from build123d import *

# Parameters (mm, degrees)
BOSS_EXTRUDE1_DEPTH = 127
SKETCH2_R           = 2.049999964
SKETCH2_W           = 19.05
SKETCH2_H           = 8.89
CUT_EXTRUDE1_DEPTH  = 25.48749992
FILLET1_R           = 12.7
BOSS_EXTRUDE2_REACH = 18.672
SKETCH4_W           = 1.891908828
SKETCH4_H           = 8.89


with BuildPart() as part:
    # Sketch1 → Boss-Extrude1 (new body)
    with BuildSketch(Plane(origin=(0, 0, 0), x_dir=(1, 0, 0), z_dir=(0, 1, 0))):
        with BuildLine():
            Line((0, 0), (-35.56, 0))
            ThreePointArc((-35.56, 0), (-39.585438943, -0.892418328), (-42.856573321, -3.402448018))
            Line((-42.856573321, -3.402448018), (-59.216961931, -22.89999992))
            Line((-59.216961931, -22.89999992), (-60.433057484, -21.87957459))
            Line((-60.433057484, -21.87957459), (-44.072668874, -2.382022687))
            ThreePointArc((-44.072668874, -2.382022687), (-40.256345434, 0.546345283), (-35.56, 1.5875))
            Line((-35.56, 1.5875), (0, 1.5875))
            Line((0, 1.5875), (0, 0))
        make_face()
    extrude(amount=BOSS_EXTRUDE1_DEPTH)

    # Sketch2 → Cut-Extrude1 (cut, through all)
    with BuildSketch(Plane(origin=(0, 0, -1.5875), x_dir=(-1, 0, 0), z_dir=(0, 0, -1))):
        with Locations((8.399999964, 88.9)):
            Circle(SKETCH2_R)
        with Locations((8.399999964, 60.116067728)):
            Circle(SKETCH2_R)
        with Locations((39.514999964, 88.9)):
            Rectangle(SKETCH2_W, SKETCH2_H)
        with Locations((39.514999964, 60.116067728)):
            Rectangle(SKETCH2_W, SKETCH2_H)
    extrude(amount=-CUT_EXTRUDE1_DEPTH, mode=Mode.SUBTRACT)

    # Fillet1
    fillet1_edges = [part.edges().sort_by_distance(p)[0] for p in [
        (0, 0, -0.79375),
        (-59.825009707, 127, 22.389787255),
        (0, 127, -0.79375),
        (-59.825009707, 0, 22.389787255),
    ]]
    fillet(fillet1_edges, radius=FILLET1_R)

    # Boss-Extrude2: up to this face of the body (flat: up to its plane)
    boss_extrude2_end = Plane(part.part.faces().sort_by_distance((-49.039999964, 88.9, 9.536713147))[0])
    # Sketch4 → Boss-Extrude2 (add, up to the picked face)
    with BuildSketch(Plane(origin=(-23.473890996, 0, -19.696933277), x_dir=(0.64278761, 0, -0.766044443), z_dir=(0.766044443, 0, 0.64278761)), mode=Mode.PRIVATE) as boss_extrude2_sk1:
        with Locations((-38.827850468, 88.9)):
            Rectangle(SKETCH4_W, SKETCH4_H)
    boss_extrude2_tool1 = split(extrude(boss_extrude2_sk1.sketch, amount=-BOSS_EXTRUDE2_REACH, mode=Mode.PRIVATE), bisect_by=boss_extrude2_end, keep=Keep.BOTH, mode=Mode.PRIVATE)
    add(boss_extrude2_tool1.solids().sort_by_distance((-48.431952, 88.9, 10.046926))[0])
    # Sketch4 → Boss-Extrude2 (add, up to the picked face)
    with BuildSketch(Plane(origin=(-23.473890996, 0, -19.696933277), x_dir=(0.64278761, 0, -0.766044443), z_dir=(0.766044443, 0, 0.64278761)), mode=Mode.PRIVATE) as boss_extrude2_sk2:
        with Locations((-38.827850468, 60.116067728)):
            Rectangle(SKETCH4_W, SKETCH4_H)
    boss_extrude2_tool2 = split(extrude(boss_extrude2_sk2.sketch, amount=-BOSS_EXTRUDE2_REACH, mode=Mode.PRIVATE), bisect_by=boss_extrude2_end, keep=Keep.BOTH, mode=Mode.PRIVATE)
    add(boss_extrude2_tool2.solids().sort_by_distance((-48.431952, 60.116068, 10.046926))[0])


solid = part.part
Verification items for the finished model (mm, model axes). A direction names the side the tool comes from. Round coordinates to 2 decimals unless told otherwise and drop trailing zeros. Write each loop counter-clockwise with the first axis right and the second up, starting at its lowest first coordinate (ties: lowest second). Pieces come first, ordered by that corner, then holes.
(1) Mould release check, pull along Y, two halves, no side actions. Record for faces 1 (the cylindrical face through (-3.82, 123.38, -0.78)), 2 (the cylindrical face through (-40.318, 27.446, -0.517)), 3 (the flat face through (-41, 55.671, 1)): pulls with the +Y half, pulls with the -Y half, needs draft (parallel to the pull), parting line crosses it, or undercut.
Returned:
face 1: pulls with the +Y half
face 2: needs draft
face 3: undercut
(2) Section check C-C (x = -8.4). Enter the section's corners in (y, z), plus the area to 3 significant figures.
Returned:
outline: (0.75, -1.59) - (58.07, -1.59) - (58.07, 0) - (0.75, 0) - close; (62.17, -1.59) - (86.85, -1.59) - (86.85, 0) - (62.17, 0) - close; (90.95, -1.59) - (126.25, -1.59) - (126.25, 0) - (90.95, 0) - close
area: 186 mm2
(3) Access from +Z, -Z, +X, -X, +Y, -Y to the whole of each face (thin tool, end or side, straight path). Record for faces 4 (the flat face through (-33.9, 0, -0.3)), 5 (the flat face through (-18, 63, 0)).
Returned:
face 4: +Z, -Z, +X, -X, -Y
face 5: +Z, +X, +Y, -Y
(4) Section check A-A (y = 88.9). Enter the section's corners in (x, z).
Returned:
outline: (-60.43, 21.88) - (-49.04, 8.3) - (-47.82, 9.32) - (-59.22, 22.9) - close; (-29.99, -1.59) - (-10.45, -1.59) - (-10.45, 0) - (-29.99, 0) - close; (-6.35, -1.59) - (0, -1.59) - (0, 0) - (-6.35, 0) - close
(5) Section check B-B (z = 5.5). Enter the section's corners in (x, y) (3 decimals).
Returned:
outline: (-46.689, 0) - (-44.617, 0) - (-44.617, 55.671) - (-46.689, 55.671) - close; (-46.689, 64.561) - (-44.617, 64.561) - (-44.617, 84.455) - (-46.689, 84.455) - close; (-46.689, 93.345) - (-44.617, 93.345) - (-44.617, 127) - (-46.689, 127) - close
(6) Depth check by flat-ended pin: pin 1 Ø1 at (x, y) = (-37.5, 52) entering from -Z; pin 2 Ø0.5 at (y, z) = (90.5, -0.5) entering from -X; pin 3 Ø5.5 at (x, z) = (-36, 4.5) entering from -Y; pin 4 Ø6 at (x, y) = (-46.5, 82.5) entering from +Z. Enter the tip coordinate at first touch or a pass-through.
Returned:
pin 1: stops at z = -1.49
pin 2: stops at x = -29.99
pin 3: passes through
pin 4: stops at z = 11.32
(7) Material ranges on line 1 (Y direction, x = -8.4, z = -0.9); line 2 (Z direction, x = -2.5, y = 94.5); line 3 (Z direction, x = -55.5, y = 28), recorded low to high.
Returned:
line 1: y = 0.75 to 58.07, 62.17 to 86.85, 90.95 to 126.25
line 2: z = -1.59 to 0
line 3: z = 16 to 18.47
